Design review of the part built by this model. Coordinates are the model's own, in mm. Face numbers are marked on the shaded views. Coordinates: 2 decimals unless noted, no trailing zeros. Write each loop counter-clockwise with the first axis right and the second up, starting at its lowest first coordinate (ties: lowest second). Pieces come first, ordered by that corner, then holes. Notation, with made-up numbers: (56, 5) - (79, 5) arc R24 cw to (79, 18) - close; hole circle Ø1 at (-6.5, 78.25). An arc over 180 degrees is marked (long way). Use a Markdown table: item, result.
from build123d import *

# Parameters (mm, degrees)
SHIELD_CROSS_SECTION_SKETCH_R   = 100
SHIELD_CROSS_SECTION_SKETCH_R_2 = 97
SHIELD_EXTRUDE_DEPTH            = 80
TOP_FILLET_R                    = 1.5
BOTTOM_FILLET_R                 = 1.5


with BuildPart() as part:
    # Shield Cross Section Sketch → Shield Extrude (new body)
    with BuildSketch(Plane(origin=(0, 0, 0), x_dir=(1, 0, 0), z_dir=(0, 1, 0))):
        with Locations(Location((0, 0, 0), (0, 0, 270))):
            Circle(SHIELD_CROSS_SECTION_SKETCH_R)
        with Locations(Location((0, 0, 0), (0, 0, 270))):
            Circle(SHIELD_CROSS_SECTION_SKETCH_R_2, mode=Mode.SUBTRACT)
    extrude(amount=SHIELD_EXTRUDE_DEPTH)

    # Top Fillet
    top_fillet_edges = [part.edges().sort_by_distance(p)[0] for p in [
        (0, 80, -100),
        (0, 80, -97),
    ]]
    fillet(top_fillet_edges, radius=TOP_FILLET_R - 0.0001)  # a hair under: the kernel refuses the full size

    # Bottom Fillet
    bottom_fillet_edges = [part.edges().sort_by_distance(p)[0] for p in [
        (0, 0, -100),
        (0, 0, -97),
    ]]
    fillet(bottom_fillet_edges, radius=BOTTOM_FILLET_R - 0.0001)  # a hair under: the kernel refuses the full size


solid = part.part
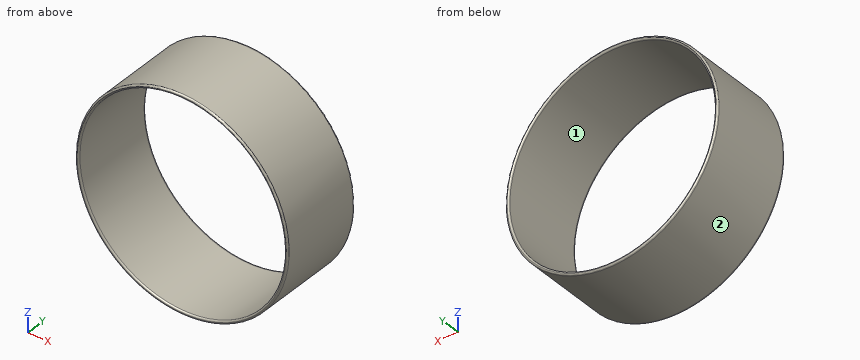
(1) For pin 1 (2 mm diameter, centred on y = 18, z = -68.5, fed in from +X); pin 2 (3 mm diameter, centred on y = 13.5, z = 58.5, fed in from +X); pin 3 (10 mm diameter, centred on y = 30, z = 71, fed in from -X), all flat-tipped, find the tip position at first contact; note any pin that passes through.
Determined:
| item | result |
|---|---|
| pin 1 | x = 73.78 |
| pin 2 | x = 82.16 |
| pin 3 | x = -75.13 |
(2) Draft analysis for pull direction X (two halves, no side actions). For the marked faces 1 and 2, state which applies: +X half, -X half, draft (parallel to the pull), parting line (faces both ways), or undercut.
Determined:
| item | result |
|---|---|
| face 1 | undercut |
| face 2 | parting line |
(3) For L1, parallel to X at y = 61.5, z = -0.5; L2, parallel to Y at x = 91.5, z = -36; L3, parallel to X at y = 24, z = 33, list the stretches that pass through material, from the lowest coordinate up. Write a range as from..to.
Determined:
| item | result |
|---|---|
| L1 | -100..-97, 97..100 |
| L2 | 0.01..79.99 |
| L3 | -94.4..-91.21, 91.21..94.4 |
(4) Take a section at C-C on y = 54. Write out the cut boundary in (x, z).
Determined:
| item | result |
|---|---|
| outline | circle Ø200 at (0, 0); hole circle Ø194 at (0, 0) |
